For this review, take the finished solid that the model builds, in its own axes (mm). Coordinates: 2 decimals unless noted, no trailing zeros. Write each loop counter-clockwise with the first axis right and the second up, starting at its lowest first coordinate (ties: lowest second). Pieces come first, ordered by that corner, then holes. Notation, with made-up numbers: (-9.75, 50.25) -> (47.25, 50.25) arc R16 cw to (47.25, 72.25) -> close; hole circle Ø2 at (77, -17.5). An arc over 180 degrees is marked (long way). Put each result on its own line as item: value. Start each with the question number.
Item 1: Consider section D-D on z = -10.16. Give the boundary of the cut face in (x, y).
Item 2: Insertion check: P1, Ø0.8, axis at x = -31.5, y = 0.5, coming from the -Z side. The pin has a flat end and moves straight along its axis. Give the tip position at first contact, or say it passes through.
Item 3: Consider section A-A on z = 22.86. Give the boundary of the cut face in (x, y), and give its area (3 significant figures).
Item 4: To check wall thickness, follow L1, parallel to X at y = 1.4, z = -17; L2, parallel to X at y = 0.6, z = -11; L3, parallel to Z at x = -22.5, y = 0.9. State the ranges of each line that lie inside material, in increasing order.
Item 5: Consider section B-B on z = -21.59. Give the boundary of the cut face in (x, y).
Item 6: Consider section C-C on y = 0.7. Give the boundary of the cut face in (x, z).
```python
from build123d import *

# Parameters (mm, degrees)
SKETCH1_W                  = 130.175
SKETCH1_H                  = 50.8
BOSS_EXTRUDE1_DEPTH        = 1.524
CUT_EXTRUDE1_REACH         = 71.885
SKETCH6_W                  = 111.125
SKETCH6_H                  = 12.7
CHAMFER2_SIZE              = 2.54
F_3_2_3_2_DIAMETER_HOLE1_D = 3.2


with BuildPart() as part:
    # Sketch1 → Boss-Extrude1 (new body)
    with BuildSketch(Plane(origin=(0, 0, 0), x_dir=(1, 0, 0), z_dir=(0, 1, 0))):
        Rectangle(SKETCH1_W, SKETCH1_H)
    extrude(amount=BOSS_EXTRUDE1_DEPTH)

    # Sketch6 → Cut-Extrude1 (cut, up to next)
    with BuildSketch(Plane(origin=(0, 1.524, 0), x_dir=(1, 0, 0), z_dir=(0, 1, 0)), mode=Mode.PRIVATE) as cut_extrude1_sk1:
        with Locations((-9.525, 19.05)):
            Rectangle(SKETCH6_W, SKETCH6_H)
    cut_extrude1_tool1 = extrude(cut_extrude1_sk1.sketch, amount=-CUT_EXTRUDE1_REACH, mode=Mode.PRIVATE) & part.part
    add(cut_extrude1_tool1.solids().sort_by_distance((-9.525, 1.524, -19.05))[0], mode=Mode.SUBTRACT)

    # Chamfer2
    chamfer2_edges = [part.edges().sort_by_distance(p)[0] for p in [
        (46.0375, 0.762, -12.7),
    ]]
    chamfer(chamfer2_edges, length=CHAMFER2_SIZE)

    # Ø3.2 (3.2) Diameter Hole1 (through all)
    with Locations(Plane(origin=(0, 1.524, 0), x_dir=(-1, 0, 0), z_dir=(0, 1, 0))):
        with Locations((-62.5475, 22.86), (-62.5475, -21.59), (-34.6075, 22.86), (-34.6075, -10.16), (61.9125, 22.86), (61.9125, -10.16)):
            Hole(F_3_2_3_2_DIAMETER_HOLE1_D / 2)


solid = part.part
```
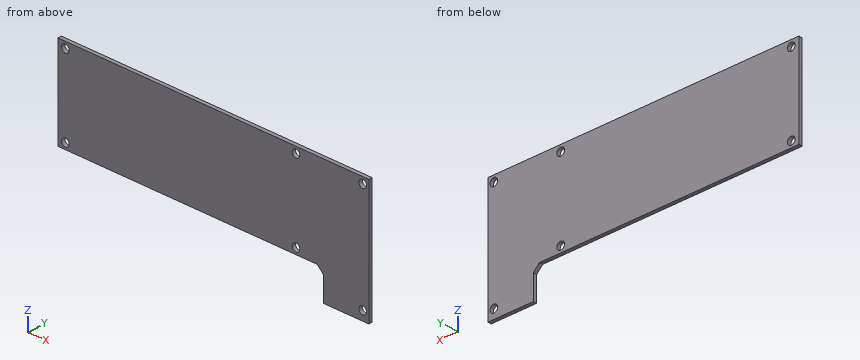
Return value:
1. outline: (-65.09, 0) -> (-63.51, 0) -> (-63.51, 1.52) -> (-65.09, 1.52) -> close; (-60.31, 0) -> (33.01, 0) -> (33.01, 1.52) -> (-60.31, 1.52) -> close; (36.21, 0) -> (65.09, 0) -> (65.09, 1.52) -> (36.21, 1.52) -> close
2. P1: z = -12.7
3. outline: (-65.09, 0) -> (-63.51, 0) -> (-63.51, 1.52) -> (-65.09, 1.52) -> close; (-60.31, 0) -> (33.01, 0) -> (33.01, 1.52) -> (-60.31, 1.52) -> close; (36.21, 0) -> (60.95, 0) -> (60.95, 1.52) -> (36.21, 1.52) -> close; (64.15, 0) -> (65.09, 0) -> (65.09, 1.52) -> (64.15, 1.52) -> close
3. area: 184 mm^2
4. L1: 46.04 to 65.09
4. L2: -65.09 to -63.27, -60.55 to 33.25, 35.97 to 65.09
4. L3: -12.7 to 25.4
5. outline: (46.04, 0) -> (60.95, 0) -> (60.95, 1.52) -> (46.04, 1.52) -> close; (64.15, 0) -> (65.09, 0) -> (65.09, 1.52) -> (64.15, 1.52) -> close
6. outline: (-65.09, -12.7) -> (43.5, -12.7) -> (46.04, -15.24) -> (46.04, -25.4) -> (65.09, -25.4) -> (65.09, 25.4) -> (-65.09, 25.4) -> close; hole circle Ø3.2 at (-61.91, -10.16); hole circle Ø3.2 at (-61.91, 22.86); hole circle Ø3.2 at (34.61, -10.16); hole circle Ø3.2 at (34.61, 22.86); hole circle Ø3.2 at (62.55, -21.59); hole circle Ø3.2 at (62.55, 22.86)
